The listing builds one solid part. Answer for the finished solid, in the listing's coordinates (mm). A direction names the side the tool comes from. Round coordinates to 2 decimals unless told otherwise and drop trailing zeros. Write each loop counter-clockwise with the first axis right and the second up, starting at its lowest first coordinate (ties: lowest second). Pieces come first, ordered by that corner, then holes.
(1) For faces 4 (the face through (224.51, 3.45, -158.48)), 5 (the face through (4, 0, 4)), determine the directions among +Z, -Z, +X, -X, +Y, -Y from which every point of the face is accessible in a straight line to the end or side of a thin tool.
(2) Find the intervals of material crossed by probe 1 along X at (y, z) = (1.25, -112); probe 2 along X at (y, z) = (4.25, -267.5); probe 3 along X at (y, z) = (1, -166), in increasing order.
(3) Each of these flat-tipped pins is pushed along its axis until it touches: pin 1 Ø3.5 at (x, y) = (-268, 2.5) entering from +Z; pin 2 Ø2 at (x, y) = (-267.5, 4) entering from -Z; pin 3 Ø4 at (x, y) = (-183, 2) entering from -Z. Where does it stop, or does it pass through?
(4) The mould has two halves that part along Z. Classify faces 1 (the face through (4, 7, 4)), 2 (the face through (224.85, 3.45, 158.73)), 3 (the face through (39.054, 3.451, -297.447)): +Z half, -Z half, draft (parallel to the pull), parting line (faces both ways), or undercut.
(5) A cutting plane is placed at C-C, the plane x = -115. Give the vertices of the cut face in (y, z).
(6) A cutting plane is placed at A-A, the plane y = 2.25. Give the number of separate pieces and of enclosed holes in the cut face, and give its area (4 significant figures).
(7) A cutting plane is placed at B-B, the plane z = 72. Give the vertices of the cut face in (x, y).
Autodesk Inventor part; units mm, degrees
ref_plane "YZ Plane" through (0, 0, 0) normal (1, 0, 0) x (0, 1, 0)
ref_plane "XZ Plane" through (0, 0, 0) normal (0, 1, 0) x (-1, 0, 0)
ref_plane "XY Plane" through (0, 0, 0) normal (0, 0, 1) x (1, 0, 0)
sketch "Sketch1" plane through (0, 0, 0) normal (0, 1, 0) x (-1, 0, 0)
  circle A0 centre (0, 0) radius 300
  line L0 (290, 3.75) -> (260, 3.75)
  line L1 (260, -3.75) -> (290, -3.75)
  arc A1 (291.75, 2) -> (290, 3.75) centre (290, 2) ccw
  arc A2 (290, -3.75) -> (291.75, -2) centre (290, -2) ccw
  arc A3 (258.25, -2) -> (260, -3.75) centre (260, -2) ccw
  arc A4 (260, 3.75) -> (258.25, 2) centre (260, 2) ccw
  line L2 (258.25, 2) -> (258.25, -2)
  line L3 (291.75, -2) -> (291.75, 2)
  line L4 (306.241, 0) -> (300, 0)
  line L5 (300, 0) -> (281.7438, 0)
  line L6 (86.0485, 276.9652) -> (76.778, 248.4335)
  arc A5 (88.2536, 278.0888) -> (86.0485, 276.9652) centre (87.7128, 276.4244) ccw
  line L7 (92.0578, 276.8527) -> (88.2536, 278.0888)
  line L8 (83.9109, 246.1159) -> (93.1814, 274.6476)
  arc A6 (93.1814, 274.6476) -> (92.0578, 276.8527) centre (91.517, 275.1884) ccw
  arc A7 (76.778, 248.4335) -> (77.9015, 246.2284) centre (78.4423, 247.8927) ccw
  line L9 (77.9015, 246.2284) -> (81.7058, 244.9923)
  arc A8 (81.7058, 244.9923) -> (83.9109, 246.1159) centre (82.2465, 246.6567) ccw
  line L10 (-236.8191, 167.4239) -> (-212.5486, 149.7904)
  arc A9 (-237.2063, 169.8683) -> (-236.8191, 167.4239) centre (-235.7905, 168.8397) ccw
  line L11 (-234.8551, 173.1044) -> (-237.2063, 169.8683)
  line L12 (-208.1402, 155.858) -> (-232.4107, 173.4915)
  arc A10 (-232.4107, 173.4915) -> (-234.8551, 173.1044) centre (-233.4394, 172.0758) ccw
  arc A11 (-212.5486, 149.7904) -> (-210.1042, 150.1775) centre (-211.52, 151.2061) ccw
  line L13 (-210.1042, 150.1775) -> (-207.7531, 153.4136)
  arc A12 (-207.7531, 153.4136) -> (-208.1402, 155.858) centre (-209.1688, 154.4422) ccw
  line L14 (-232.4107, -173.4915) -> (-208.1402, -155.858)
  arc A13 (-234.8551, -173.1044) -> (-232.4107, -173.4915) centre (-233.4394, -172.0758) ccw
  line L15 (-237.2063, -169.8683) -> (-234.8551, -173.1044)
  line L16 (-212.5486, -149.7904) -> (-236.8191, -167.4239)
  arc A14 (-236.8191, -167.4239) -> (-237.2063, -169.8683) centre (-235.7905, -168.8397) ccw
  arc A15 (-208.1402, -155.858) -> (-207.7531, -153.4136) centre (-209.1688, -154.4422) ccw
  line L17 (-207.7531, -153.4136) -> (-210.1042, -150.1775)
  arc A16 (-210.1042, -150.1775) -> (-212.5486, -149.7904) centre (-211.52, -151.2061) ccw
  line L18 (93.1814, -274.6476) -> (83.9109, -246.1159)
  arc A17 (92.0578, -276.8527) -> (93.1814, -274.6476) centre (91.517, -275.1884) ccw
  line L19 (88.2536, -278.0888) -> (92.0578, -276.8527)
  line L20 (76.778, -248.4335) -> (86.0485, -276.9652)
  arc A18 (86.0485, -276.9652) -> (88.2536, -278.0888) centre (87.7128, -276.4244) ccw
  arc A19 (83.9109, -246.1159) -> (81.7058, -244.9923) centre (82.2465, -246.6567) ccw
  line L21 (81.7058, -244.9923) -> (77.9015, -246.2284)
  arc A20 (77.9015, -246.2284) -> (76.778, -248.4335) centre (78.4423, -247.8927) ccw
  point P0 (87.0636, 267.9543)
  point P1 (-227.9355, 165.6049)
  point P2 (-227.9355, -165.6049)
  point P3 (87.0636, -267.9543)
  dimension "d3" = 7.5
  dimension "d6" = 30
  dimension "d7" = 3.5
  dimension "d8" = 3.5
  dimension "d26" = 8.25
  dimension "d27" = 33.5
  dimension "d28" = 7.5
extrude "Extrusion1" add sketch "Sketch1" along normal blind 7
properties part number "Roof - V2"
Solutions:
1. face 4: +Y, -Y
1. face 5: +Z, -Z, +X, -X, -Y
2. probe 1: x = -278.31 to 278.31
2. probe 2: x = -135.81 to -90.86, -82.97 to 135.81
2. probe 3: x = -249.89 to 222.1, 234.86 to 249.89
3. pin 1: stops at z = 138.24
3. pin 2: stops at z = -137.76
3. pin 3: stops at z = -239.25
4. face 1: draft
4. face 2: undercut
4. face 3: parting line
5. outline: (0, -277.08) - (7, -277.08) - (7, 277.08) - (0, 277.08) - close
6. separate pieces: 1
6. enclosed holes: 5
6. area: 281,500 mm2
7. outline: (-291.23, 0) - (291.23, 0) - (291.23, 7) - (-291.23, 7) - close
